Model file for the job. Use its own axes, mm. Coordinates: 2 decimals unless noted, no trailing zeros. One line per question, with ' | ' between items. Start each with the question number.
(1) Flat gauge pin, fed straight in: pin 1 Ø4 at (x, z) = (-14.52, -127.45) entering from +Y. Where does the tip first touch, or does it go through?
(2) Two-plate mould, pull along X, no slides. Class faces 1 (the face through (-14.22, 0.783, -129.743)), 2 (the face through (4.321, 0.792, 137.315)), 3 (the face through (4.58, 0.79, -134.69)): +X half, -X half, draft (parallel to the pull), parting line (faces both ways), or undercut.
(3) Wall check: probe 1 along X at (y, z) = (1.1, -73.5); probe 2 along Z at (x, y) = (-15, 0.8); probe 3 along Z at (x, y) = (-12.5, 1). Give the ranges that are in metal, low to high.
Autodesk Inventor part; units mm, degrees
ref_plane "YZ Plane" through (0, 0, 0) normal (1, 0, 0) x (0, 1, 0)
ref_plane "XZ Plane" through (0, 0, 0) normal (0, 1, 0) x (-1, 0, 0)
ref_plane "XY Plane" through (0, 0, 0) normal (0, 0, 1) x (1, 0, 0)
sketch "Sketch1" plane through (0, 0, 0) normal (0, 1, 0) x (-1, 0, 0)
  line L0 (27.8561, -123.3839) -> (27.8561, 130.6161)
  line L1 (27.8561, 130.6161) -> (-35.6439, 130.6161) construction
  line L2 (-35.6439, 130.6161) -> (-35.6439, -123.3839)
  line L3 (27.8561, -146.496) -> (-35.6439, -123.3839)
  line L4 (27.8561, -146.496) -> (27.8561, -123.3839)
  arc A0 (27.8561, 130.6161) -> (-35.6439, 130.6161) centre (-3.8939, 58.7362) ccw
  line L5 (-35.6439, -123.3839) -> (-3.8939, -52.0908)
  point P0 (0, 0)
  dimension "d3" = 254
  dimension "d4" = 110
  dimension "d6" = 78.5798
  dimension "d24" = 24.006
extrude "Extrusion1" add sketch "Sketch1" along normal blind 1.5875
fillet "Fillet1" radius 3.175 4 edges at (-27.8561, 0.7937, -146.496) (35.6439, 0.7937, -123.3839) (35.6439, 0.7937, 130.6161) (-27.8561, 0.7937, 130.6161)
fillet "Fillet2" radius 0.635 16 edges at (-27.3175, 1.5875, 130.2862) (3.8939, 1.5875, 137.316) (35.1052, 1.5875, 130.2862) (35.6439, 1.5875, 3.6781) (35.0697, 1.5875, -122.9818) (4.9798, 1.5875, -134.5447) (-26.5022, 1.5875, -144.5624) (-27.8561, 1.5875, 2.5665) (-26.5022, 0, -144.5624) (4.9798, 0, -134.5447) (35.0697, 0, -122.9818) (35.6439, 0, 3.6781) (35.1052, 0, 130.2862) (3.8939, 0, 137.316) (-27.3175, 0, 130.2862) (-27.8561, 0, 2.5665)
sketch "Sketch3" plane through (0, 0, 0) normal (0, -1, 0) x (1, 0, 0)
  circle A0 centre (10.8789, -105.1316) radius 2.3114
  circle A1 centre (-14.5211, -117.8316) radius 2.3114
  circle A2 centre (23.5789, -105.1316) radius 2.3114
  arc A3 (-27.2211, -141.9616) -> (-23.8124, -144.3485) centre (-24.6811, -141.9616) ccw
  line L0 (33.3376, -123.5476) -> (-23.8124, -144.3485)
  arc A4 (33.3376, -123.5476) -> (35.0089, -121.1607) centre (32.4689, -121.1607) ccw
  line L1 (35.0089, 128.5169) -> (35.0089, -121.1607)
  arc A5 (35.0089, 128.5169) -> (33.4314, 130.8675) centre (32.4689, 128.5169) ccw
  arc A6 (33.4314, 130.8675) -> (-25.6437, 130.8675) centre (3.8939, 58.7362) ccw
  arc A7 (-25.6437, 130.8675) -> (-27.2211, 128.5169) centre (-24.6811, 128.5169) ccw
  line L2 (-27.2211, -141.9616) -> (-27.2211, 128.5169)
  line L3 (32.4689, -121.1607) -> (15.1752, -73.6466)
  point P0 (0, 0)
  dimension "d39" = 20
sketch "Sketch4" plane through (0, 0, 0) normal (0, -1, 0) x (0.9397, 0, 0.342)
  line L0 (-10.9286, -127.4989) -> (-71.7464, -127.4989)
  line L1 (-74.1332, -124.0901) -> (18.3759, 130.0766)
  circle A0 centre (-57.2364, -114.7989) radius 2.3114
  line L2 (-10.9286, -124.9589) -> (-10.9286, -74.3954) construction
  line L3 (-10.9286, -124.9589) -> (-35.7001, -124.9589) construction
  circle A1 centre (-57.2364, -102.0989) radius 2.3114
  circle A2 centre (-57.2364, -89.3989) radius 2.3114
  circle A3 centre (-44.5364, -114.7989) radius 2.3114
  circle A4 centre (-44.5364, -102.0989) radius 2.3114
  circle A5 centre (-44.5364, -89.3989) radius 2.3114
  circle A6 centre (-31.8364, -114.7989) radius 2.3114
  circle A7 centre (-31.8364, -102.0989) radius 2.3114
  circle A8 centre (-31.8364, -89.3989) radius 2.3114
  circle A9 centre (-19.1364, -114.7989) radius 2.3114
  circle A10 centre (-19.1364, -102.0989) radius 2.3114
  circle A11 centre (-19.1364, -89.3989) radius 2.3114
  circle A12 centre (-6.4364, -114.7989) radius 2.3114
  circle A13 centre (-6.4364, -102.0989) radius 2.3114
  circle A14 centre (-6.4364, -89.3989) radius 2.3114
  point P0 (0, 0)
  dimension "d26" = 4.6228
  dimension "d27" = 12.7
  dimension "d28" = 12.7
  dimension "d31" = 12.7
  dimension "d34" = 12.7
extrude "Extrusion3" cut sketch "Sketch4" against normal blind 25.4 contours A0 | A7 | A10
properties part number "large ball holder"
Filled in:
1) pin 1: through
2) face 1: undercut | face 2: parting line | face 3: +X half
3) probe 1: -27.84 to 35.63 | probe 2: -141.82 to -129.71, -125.19 to 135.01 | probe 3: -140.9 to -128.57, -126.33 to 135.59
